Geometry: final body of the model. Coordinates: model frame, mm. A direction names the side the tool comes from. Coordinates: 2 decimals unless noted, no trailing zeros. Write each loop counter-clockwise with the first axis right and the second up, starting at its lowest first coordinate (ties: lowest second). Pieces come first, ordered by that corner, then holes. Notation, with made-up numbers: (59.5, 21) - (63.5, 21) arc R18 ccw to (63.5, 31) - close; hole circle Ø5 at (22.25, 24). An arc over 180 degrees is marked (long way). Answer as a JSON object with one key per item and string values. Group by question number.
Item 1: First-contact query: pin 1 Ø4 at (x, y) = (-5, 3) entering from -Z; pin 2 Ø2 at (x, y) = (5, 1.5) entering from -Z; pin 3 Ø5 at (y, z) = (8.5, -10.5) entering from +X. Flat tips, straight axial feed; report the tip coordinate or a pass-through.
Item 2: Line query: line 1 along X through (y, z) = (9.5, 0); line 2 along Z through (x, y) = (-0.75, 1.5); line 3 along X through (y, z) = (10.25, 1.75). Output: solid intervals per line, ascending. Write a range as from..to.
Item 3: Section B-B on y = 8. Return loops of the section in (x, z).
Item 4: Set-up query: faces 4 (the flat face through (0, 12, 0)), 5 (the cylindrical face through (0.66, 5.916, -14.985)). Return all of +Z, -Z, +X, -X, +Y, -Y with unobstructed straight access to the full face (end or side cutting, diameter ignored); none if empty.
Item 5: Section C-C on x = -0.5. Return loops of the section in (y, z).
Item 6: Section D-D on z = 0. Return loops of the section in (x, y), and give its area (3 significant figures).
Item 7: Mould query, pull axis Z, two halves, no side actions, for faces 1 (the flat face through (10, 12, -7)), 2 (the cylindrical face through (-1.119, 5.916, 2.998)), 3 (the cylindrical face through (3.604, 13.479, 11.446)). Classes: pulls with the +Z half, pulls with the -Z half, needs draft (parallel to the pull), parting line crosses it, or undercut.
Item 8: Section A-A on z = -10.75. Return loops of the section in (x, y).
```python
from build123d import *

# Parameters (mm, degrees)
SKETCH1_R           = 15
BOSS_EXTRUDE1_DEPTH = 12
SKETCH2_R           = 12
BOSS_EXTRUDE2_DEPTH = 3


with BuildPart() as part:
    # Sketch1 → Boss-Extrude1 (new body)
    with BuildSketch(Plane(origin=(0, 0, 0), x_dir=(1, 0, 0), z_dir=(0, 1, 0))):
        with Locations(Location((0, 0, 0), (0, 0, 270))):
            Circle(SKETCH1_R)
        with BuildLine():
            Line((-0.965663189, 3.050818678), (2.836784234, 1.480761699))
            ThreePointArc((2.836784234, 1.480761699), (-1.221287526, -2.957779028), (-0.965663189, 3.050818678))
        make_face(mode=Mode.SUBTRACT)
    extrude(amount=BOSS_EXTRUDE1_DEPTH)

    # Sketch2 → Boss-Extrude2 (add)
    with BuildSketch(Plane(origin=(0, 12, 0), x_dir=(1, 0, 0), z_dir=(0, 1, 0))):
        with Locations(Location((0, 0, 0), (0, 0, 270))):
            Circle(SKETCH2_R)
    extrude(amount=BOSS_EXTRUDE2_DEPTH)


solid = part.part
```
Checks:
{
 "1": {"pin 1": "z = -14.7", "pin 2": "z = -14.46", "pin 3": "x = 12.69"},
 "2": {"line 1": "-15..-3.2, 3.2..15", "line 2": "-14.98..-2.96, 3.11..14.98", "line 3": "-14.9..-2.68, 2.68..14.9"},
 "3": {"outline": "circle Ø30 at (0, 0); hole (-0.97, -3.05) - (2.84, -1.48) arc R3.2 ccw (long way) to start"},
 "4": {"face 4": "-Y", "face 5": "+Y, -Y"},
 "5": {"outline": "(0, -14.99) - (12, -14.99) - (12, -11.99) - (15, -11.99) - (15, 11.99) - (12, 11.99) - (12, 14.99) - (0, 14.99) - (0, 3.16) - (12, 3.16) - (12, -2.86) - (0, -2.86) - close"},
 "6": {"outline": "(-15, 0) - (-3.2, 0) - (-3.2, 12) - (3.2, 12) - (3.2, 0) - (15, 0) - (15, 12) - (12, 12) - (12, 15) - (-12, 15) - (-12, 12) - (-15, 12) - close", "area": "355 mm^2"},
 "7": {"face 1": "needs draft", "face 2": "undercut", "face 3": "parting line crosses it"},
 "8": {"outline": "(-10.46, 0) - (10.46, 0) - (10.46, 12) - (5.33, 12) - (5.33, 15) - (-5.33, 15) - (-5.33, 12) - (-10.46, 12) - close"}
}
